Part model, mm, in its own coordinate system. Face numbers are marked on the shaded views. A direction names the side the tool comes from. Coordinates: 2 decimals unless noted, no trailing zeros. Loops run counter-clockwise (first coordinate to the right, second up) from the corner with the lowest first, then second, coordinate; pieces in that order, holes last. Notation, with made-up numbers: (88, 75.25) -> (97, 75.25) arc R23 ccw to (97, 92.25) -> close; hole circle Ø8 at (62.5, 80). An arc over 180 degrees is marked (long way). One line per question, with ' | ' between items. Start each with the question number.
1) 3-axis set-ups, long thin cutter, end or side, ignore diameter. For the marked faces 5 and 6: which of +Z, -Z, +X, -X, +Y, -Y reach the whole face in a straight line?
2) Cut at C-C (x = 6.5). List the corners of the cut face in (y, z).
3) Cut at A-A (z = -3.5). List the corners of the cut face in (x, y).
4) Two-plate mould, pull along X, no slides. Class the marked faces 1, 2, 3 and 4: released by +X, released by -X, zero draft, split by the parting line, or undercut.
5) Cut at B-B (y = -38.5). List the corners of the cut face in (x, z), plus the area to 3 significant figures.
6) Probe L1, parallel to Z at x = -38.5, y = -46.5; L2, parallel to X at y = -42, z = -26.5; L3, parallel to Z at x = -42, y = -81.5. List the from-to ranges inside material, lowest first. Write a range as from..to.
7) Drop flat-ended pins along their axis: pin 1 (1 mm diameter, centred on x = -51, y = -17, fed in from -Z); pin 2 (5 mm diameter, centred on x = -50.5, z = 10, fed in from +Y). Give the stop position or say it passes through.
8) Cut at D-D (z = -41). List the corners of the cut face in (x, y).
from build123d import *

# Parameters (mm, degrees)
F0_W     = 100.477673
F0_H     = 100.787793
F1_DEPTH = 100
F2_SIZE  = 25
F3_SIZE  = 25
F5_DEPTH = 100


with BuildPart() as f1:
    # F0 (on Front) → F1 (new body)
    with BuildSketch(Plane.XZ):
        with Locations((-14.575462, -13.490057)):
            Rectangle(F0_W, F0_H)
    extrude(amount=F1_DEPTH)

    # F2
    f2_edges = [f1.edges().sort_by_distance(p)[0] for p in [
        (35.663374, -50, 36.90384),
    ]]
    chamfer(f2_edges, length=F2_SIZE)

    # F3
    f3_edges = [f1.edges().sort_by_distance(p)[0] for p in [
        (-64.814299, -50, -63.883953),
    ]]
    chamfer(f3_edges, length=F3_SIZE)

    # F4 (on face) → F5 (cut)
    with BuildSketch(Plane.XZ.offset(100)):
        Polygon((-42.732559, 22.58721), (-42.732559, -38.154069), (8.241279, -9.767442), align=None)
    extrude(amount=-F5_DEPTH, mode=Mode.SUBTRACT)


solid = f1.part
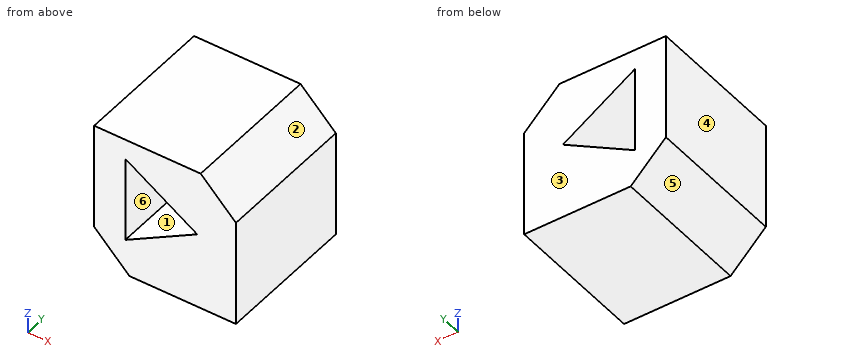
Reported:
1) face 5: -Z, -X, +Y, -Y | face 6: +Y, -Y
2) outline: (-100, -63.88) -> (0, -63.88) -> (0, -10.74) -> (-100, -10.74) -> close; (-100, -8.66) -> (0, -8.66) -> (0, 36.9) -> (-100, 36.9) -> close
3) outline: (-64.81, -100) -> (-42.73, -100) -> (-42.73, 0) -> (-64.81, 0) -> close; (-1.63, -100) -> (35.66, -100) -> (35.66, 0) -> (-1.63, 0) -> close
4) face 1: undercut | face 2: released by +X | face 3: zero draft | face 4: released by -X
5) outline: (-64.81, -38.88) -> (-39.81, -63.88) -> (35.66, -63.88) -> (35.66, 11.9) -> (10.66, 36.9) -> (-64.81, 36.9) -> close; hole (-42.73, -38.15) -> (8.24, -9.77) -> (-42.73, 22.59) -> close | area: 7,950 mm²
6) L1: z = -63.88..-35.8, 19.9..36.9 | L2: x = -64.81..-42.73, -21.81..35.66 | L3: z = -61.7..-37.75, 22.12..36.9
7) pin 1: stops at z = -53.2 | pin 2: stops at y = 0
8) outline: (-62.7, -100) -> (35.66, -100) -> (35.66, 0) -> (-62.7, 0) -> close
